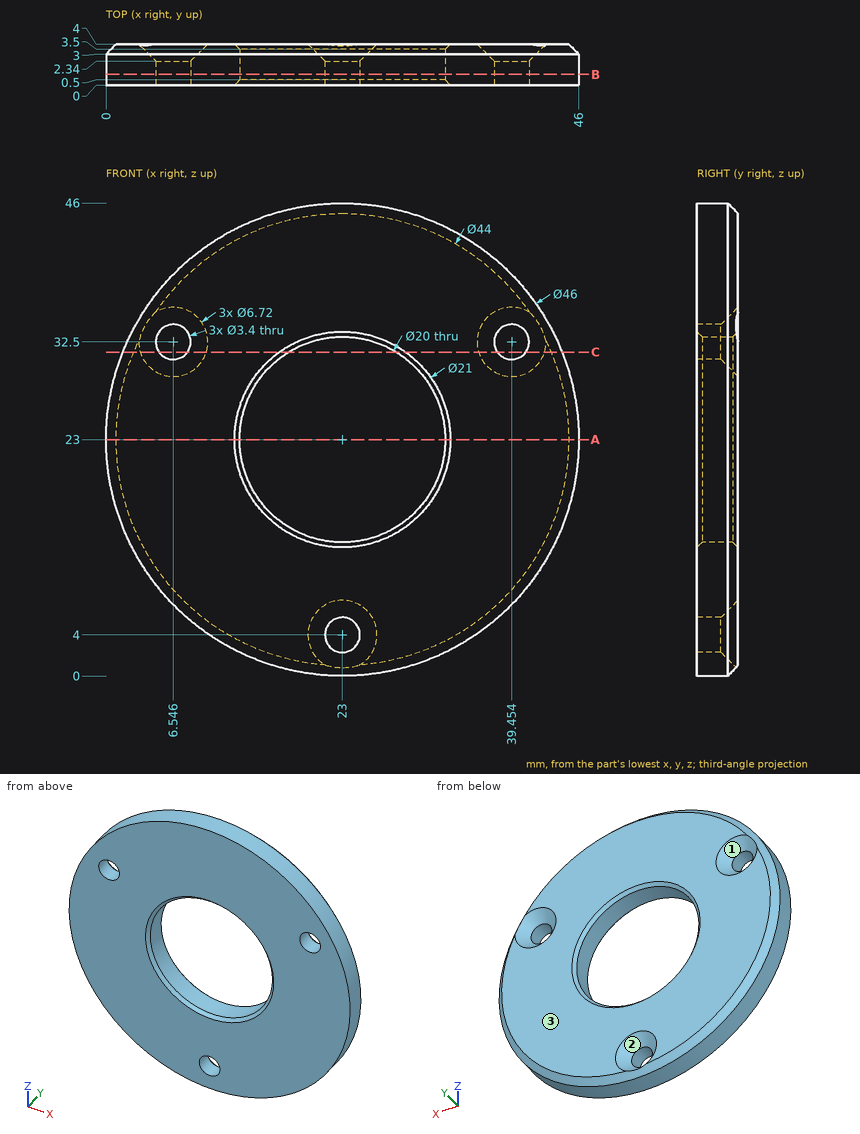
Study the drawing (mm; zero at the part's minimum x, y, z) and answer. Round coordinates to 2 decimals unless told otherwise and drop trailing zeros. Write each loop counter-clockwise with the first axis right and the second up, starting at its lowest first coordinate (ties: lowest second). Pieces come first, ordered by that corner, then holes. Notation, with made-up numbers: (81, 87.5) - (129, 87.5) arc R32 cw to (129, 123.5) - close; hole circle Ø5 at (18.25, 7.5). An arc over 180 degrees is marked (long way). Return JSON: item names as keys, results as strings. Group by question number.
Q1. The part is cut by section C-C on z = 31.5. Count the separate pieces of the cut face and the enclosed holes in it.
Q2. The part is cut by section B-B on y = 1.05. Write down the section's boundary in (x, z) (1 decimal), then the cut area to 3 significant figures.
Q3. Each of these flat-tipped pins is pushed along its axis until it touches: pin 1 Ø2 at (x, z) = (18.5, 15) entering from -Y; pin 2 Ø1 at (x, y) = (24, 2) entering from +Z (1 decimal); pin 3 Ø1.5 at (x, y) = (13, 2) entering from +Z. Where does it stop, or does it pass through?
Q4. Find the intervals of material crossed by L1, parallel to X at y = 1.9, z = 23; L2, parallel to X at y = 1.4, z = 32 (1 decimal); L3, parallel to Z at x = 6.5, y = 3.6, in increasing order.
Q5. The mould has two halves that part along Z. Classify the marked faces 1, 2 and 3: released by +Z, released by -Z, zero draft, split by the parting line, or undercut.
Q6. The part is cut by section A-A on z = 23. Write down the section's boundary in (x, y).
Solved:
{
 "1": {"separate pieces": "4", "enclosed holes": "0"},
 "2": {"outline": "circle Ø46 at (23, 23); hole circle Ø3.4 at (6.5, 32.5); hole circle Ø20 at (23, 23); hole circle Ø3.4 at (23, 4); hole circle Ø3.4 at (39.5, 32.5)", "area": "1,320 mm²"},
 "3": {"pin 1": "y = 0.32", "pin 2": "z = 46", "pin 3": "z = 44.06"},
 "4": {"L1": "0 to 13, 33 to 46", "L2": "1.8 to 4.9, 8.2 to 18.6, 27.4 to 37.8, 41.1 to 44.2", "L3": "7.85 to 29.54, 35.46 to 38.15"},
 "5": {"face 1": "undercut", "face 2": "undercut", "face 3": "zero draft"},
 "6": {"outline": "(0, 0) - (12.5, 0) - (13, 0.5) - (13, 3.5) - (12.5, 4) - (1, 4) - (0, 3) - close; (33, 0.5) - (33.5, 0) - (46, 0) - (46, 3) - (45, 4) - (33.5, 4) - (33, 3.5) - close"}
}
